Geometry check sheet. Reference: the model listing, model coordinates, mm. A direction names the side the tool comes from. Coordinates: 2 decimals unless noted, no trailing zeros. Write each loop counter-clockwise with the first axis right and the second up, starting at its lowest first coordinate (ties: lowest second). Pieces come first, ordered by that corner, then holes. Notation, with made-up numbers: M 51.5,47.25 L 109.5,47.25 A19 ccw 109.5,56.25 Z; hole C 14.25,51 d11. An arc over 180 degrees is marked long. Put each result on its own line as item: value. Start each with the question number.
1) Cross-section at B-B on x = 0. Record the cut outline in (y, z) (1 decimal).
2) Mould release check, pull along Z, two halves, no side actions. Record for faces 1 (the cylindrical face through (0.221, 1.565, 20.814)), 2 (the cylindrical face through (-8.32, 1.57, -26.41)), 3 (the flat face through (0, 3.175, 12)): released by +Z, released by -Z, zero draft, split by the parting line, or undercut.
3) Cross-section at C-C on z = 22.5. Record the cut outline in (x, y) (3 decimals).
4) Gauge pin test, flat ends, axial feed: pin 1 (22 mm diameter, centred on x = 0, z = 0, fed in from -Y); pin 2 (3 mm diameter, centred on x = 0, z = -22.5, fed in from -Y); pin 3 (1.5 mm diameter, centred on y = 2.5, z = -6, fed in from +X). Record the tip position at first contact, or that the pin passes through.
5) Cross-section at D-D on y = 1.1. Record the cut outline in (x, z).
6) Scan lines: line 1 along X through (y, z) = (1.1, 1); line 2 along Z through (x, y) = (2.5, 2.15); line 3 along X through (y, z) = (1.4, -22). Record each from-to range of solid material in increasing order.
7) Cross-section at A-A on z = 0. Record the cut outline in (x, y) (1 decimal), plus the area to 3 significant figures.
8) Set-up check for faces 4 (the cylindrical face through (-8.32, 0.8, 9.07)), 5 (the cylindrical face through (20.93, 1.57, 0.65)): record each of +Z, -Z, +X, -X, +Y, -Y from which the full face is reachable in a straight line by a thin tool's end or side.
from build123d import *

# Parameters (mm, degrees)
M3_CLEARANCE_HOLE1_D = 3.4


with BuildPart() as part:
    # Sketch1 → Revolve1 (revolve)
    with BuildSketch(Plane.XY, mode=Mode.PRIVATE) as revolve1_sk:
        Polygon((12.3063, 0), (12.3063, 1.5875), (9.906, 1.5875), (9.906, 3.175), (27.69, 3.175), (27.69, 0), align=None)
    revolve(revolve1_sk.sketch.rotate(Axis((0, 0, 0), (0, 1, 0)), 90), axis=Axis((0, 0, 0), (0, 1, 0)))

    # M3 Clearance Hole1 (through all)
    with Locations(Plane(origin=(0, 3.175, 0), x_dir=(1, 0, 0), z_dir=(0, 1, 0))):
        with Locations((22.5, 0), (0, 22.5), (-22.5, 0), (0, -22.5)):
            Hole(M3_CLEARANCE_HOLE1_D / 2)


solid = part.part
Answer key:
1. outline: M 0,-27.7 L 3.2,-27.7 L 3.2,-24.2 L 0,-24.2 Z; M 0,-20.8 L 3.2,-20.8 L 3.2,-9.9 L 1.6,-9.9 L 1.6,-12.3 L 0,-12.3 Z; M 0,12.3 L 1.6,12.3 L 1.6,9.9 L 3.2,9.9 L 3.2,20.8 L 0,20.8 Z; M 0,24.2 L 3.2,24.2 L 3.2,27.7 L 0,27.7 Z
2. face 1: undercut
2. face 2: split by the parting line
2. face 3: zero draft
3. outline: M -16.14,0 L -1.7,0 L -1.7,3.175 L -16.14,3.175 Z; M 1.7,0 L 16.14,0 L 16.14,3.175 L 1.7,3.175 Z
4. pin 1: stops at y = 1.59
4. pin 2: passes through
4. pin 3: stops at x = 27.19
5. outline: C 0,0 d55.38; hole C -22.5,0 d3.4; hole C 0,0 d24.61; hole C 0,-22.5 d3.4; hole C 0,22.5 d3.4; hole C 22.5,0 d3.4
6. line 1: x = -27.67 to -23.87, -21.13 to -12.27, 12.27 to 21.13, 23.87 to 27.67
6. line 2: z = -27.58 to -9.59, 9.59 to 27.58
6. line 3: x = -16.81 to -1.62, 1.62 to 16.81
7. outline: M -27.7,0 L -24.2,0 L -24.2,3.2 L -27.7,3.2 Z; M -20.8,0 L -12.3,0 L -12.3,1.6 L -9.9,1.6 L -9.9,3.2 L -20.8,3.2 Z; M 9.9,1.6 L 12.3,1.6 L 12.3,0 L 20.8,0 L 20.8,3.2 L 9.9,3.2 Z; M 24.2,0 L 27.7,0 L 27.7,3.2 L 24.2,3.2 Z
7. area: 83.7 mm²
8. face 4: -Y
8. face 5: +Y, -Y
